For this review, take the finished solid that the model builds, in its own axes (mm). A direction names the side the tool comes from. Coordinates: 2 decimals unless noted, no trailing zeros. Loops run counter-clockwise (first coordinate to the right, second up) from the corner with the lowest first, then second, coordinate; pieces in that order, holes last. Notation, with made-up numbers: (82.25, 68) -> (118.25, 68) arc R19 cw to (118.25, 79) -> close; hole circle Ø7 at (14, 2). An arc over 180 degrees is marked (long way). Answer in a Markdown table with one row per item.
from build123d import *

# Parameters (mm, degrees)
SKETCH_1_W          = 41
SKETCH_1_H          = 71
EXTRUDE_1_DEPTH     = 3
SKETCH_2_W          = 41
SKETCH_2_H          = 10
CUT_EXTRUDE_1_DEPTH = 0.6
HOLE_WIZARD_M41_D   = 4.5
HOLE_WIZARD_M31_D   = 3.4
HOLE_WIZARD_M32_D   = 3.4


with BuildPart() as part:
    # Эскиз1 → Бобышка-Вытянуть1 (new body)
    with BuildSketch(Plane(origin=(0, 0, 0), x_dir=(1, 0, 0), z_dir=(0, 1, 0))):
        with Locations((20.5, 35.5)):
            Rectangle(SKETCH_1_W, SKETCH_1_H)
    extrude(amount=EXTRUDE_1_DEPTH)

    # Эскиз2 → Вырез-Вытянуть1 (cut)
    with BuildSketch(Plane(origin=(0, 3, 0), x_dir=(1, 0, 0), z_dir=(0, 1, 0))):
        with Locations((20.5, 5)):
            Rectangle(SKETCH_2_W, SKETCH_2_H)
        Polygon((0, 71), (10, 71), (10, 30), (31, 30), (31, 71), (41, 71), (41, 30), (41, 20), (0, 20), (0, 30), align=None)
    extrude(amount=-CUT_EXTRUDE_1_DEPTH, mode=Mode.SUBTRACT)

    # Отверстие с зазором M41 (through all)
    with Locations(Plane(origin=(24.31748925, 3, -29.970792186), x_dir=(1, 0, 0), z_dir=(0, 1, 0))):
        with Locations((-20.297457148, -24.970792186), (12.662478647, -24.970792186), (12.662478647, -4.970792186), (-20.297457148, -4.970792186), (-19.31748925, 4.049239917), (11.68251075, 4.049239917), (11.68251075, 37.009175711), (-19.31748925, 37.009175711)):
            Hole(HOLE_WIZARD_M41_D / 2)

    # Отверстие с зазором M31 (through all)
    with Locations(Plane(origin=(24.31748925, 3, -29.970792186), x_dir=(1, 0, 0), z_dir=(0, 1, 0))):
        with Locations((-3.81748925, -24.970792186), (-3.81748925, -4.970792186), (-19.31748925, 20.529207814), (11.68251075, 20.529207814)):
            Hole(HOLE_WIZARD_M31_D / 2)

    # Отверстие с зазором M32 (through all)
    with Locations(Plane(origin=(0, 3, 0), x_dir=(1, 0, 0), z_dir=(0, 1, 0))):
        with Locations((16.257359313, 46.257359313), (16.257359313, 54.742640687), (24.742640687, 54.742640687), (24.742640687, 46.257359313)):
            Hole(HOLE_WIZARD_M32_D / 2)


solid = part.part
Item 1: Take a section at C-C, the plane z = -50.5. State the section outline as (x, y) points.
Worked answers:
| item | result |
|---|---|
| outline | (0, 0) -> (3.3, 0) -> (3.3, 2.4) -> (0, 2.4) -> close; (6.7, 0) -> (34.3, 0) -> (34.3, 2.4) -> (31, 2.4) -> (31, 3) -> (10, 3) -> (10, 2.4) -> (6.7, 2.4) -> close; (37.7, 0) -> (41, 0) -> (41, 2.4) -> (37.7, 2.4) -> close |
Item 2: Insertion check: pin 1 (5 mm diameter, centred on x = 36, z = -66.98, fed in from +Y); pin 2 (0.5 mm diameter, centred on x = 21, y = 3, fed in from +Z). Each pin has a flat end and moves straight along its axis. Give the tip position at first contact, or say it passes through.
Worked answers:
| item | result |
|---|---|
| pin 1 | y = 2.4 |
| pin 2 | z = -10 |
Item 3: Take a section at B-B, the plane x = 20.5. State the section outline as (y, z) points, and give its area (3 significant figures).
Worked answers:
| item | result |
|---|---|
| outline | (0, -71) -> (3, -71) -> (3, -30) -> (2.4, -30) -> (2.4, -26.7) -> (0, -26.7) -> close; (0, -23.3) -> (2.4, -23.3) -> (2.4, -20) -> (3, -20) -> (3, -10) -> (2.4, -10) -> (2.4, -6.7) -> (0, -6.7) -> close; (0, -3.3) -> (2.4, -3.3) -> (2.4, 0) -> (0, 0) -> close |
| area | 185 mm² |
Item 4: The part is to be moulded in two halves that separate along X. For faces 1 (the cylindrical face through (3.43, 1.18, -49.85)), 2 (the flat face through (20, 1, 0)), 3 (the flat face through (0, 1, -35)), say which applies: +X half, -X half, draft (parallel to the pull), parting line (faces both ways), or undercut.
Worked answers:
| item | result |
|---|---|
| face 1 | undercut |
| face 2 | draft |
| face 3 | -X half |
Item 5: For faces 4 (the flat face through (20, 1, -71)), 5 (the flat face through (20, 2.4, -7)), list the 3-axis set-ups (+Z, -Z, +X, -X, +Y, -Y) from which the entire face can be reached by the end or side of a thin tool; tool diameter is ignored.
Worked answers:
| item | result |
|---|---|
| face 4 | -Z, +X, -X, +Y, -Y |
| face 5 | +Z, +X, -X, +Y |
Item 6: Take a section at A-A, the plane z = -5. State the section outline as (x, y) points.
Worked answers:
| item | result |
|---|---|
| outline | (0, 0) -> (1.77, 0) -> (1.77, 2.4) -> (0, 2.4) -> close; (6.27, 0) -> (18.8, 0) -> (18.8, 2.4) -> (6.27, 2.4) -> close; (22.2, 0) -> (34.73, 0) -> (34.73, 2.4) -> (22.2, 2.4) -> close; (39.23, 0) -> (41, 0) -> (41, 2.4) -> (39.23, 2.4) -> close |
Item 7: Take a section at D-D, the plane x = 8. State the section outline as (y, z) points.
Worked answers:
| item | result |
|---|---|
| outline | (0, -71) -> (2.4, -71) -> (2.4, -20) -> (3, -20) -> (3, -10) -> (2.4, -10) -> (2.4, 0) -> (0, 0) -> close |
Item 8: For L1, parallel to X at y = 1.9, z = -25; L2, parallel to Z at x = 27.5, y = 2.6; L3, parallel to Z at x = 5, y = 1.8, list the stretches that pass through material, from the lowest coordinate up.
Worked answers:
| item | result |
|---|---|
| L1 | 0 to 1.77, 6.27 to 18.8, 22.2 to 34.73, 39.23 to 41 |
| L2 | -71 to -30, -20 to -10 |
| L3 | -71 to -69.23, -64.73 to -52.2, -48.8 to -36.27, -31.77 to -27.03, -22.97 to -7.03, -2.97 to 0 |
